Part model, mm, in its own coordinate system. Give positions to 0.01 mm unless a question says otherwise; leave off trailing zeros. Order: outer loops, then holes, each group sorted by start corner. A loop starts at its lowest first (then second) coordinate and runs counter-clockwise, first axis right, second up. Notation, with made-up numbers: (-11, 2) - (14, 2) arc R20 cw to (14, 38) - close; hole circle Ø8 at (-25.75, 89). An arc over 180 degrees is marked (long way). One line per item, written item: value.
```python
from build123d import *

# Parameters (mm, degrees)
CIRPATTERN1_COUNT = 2
CIRPATTERN1_ANGLE = 90


with BuildPart() as part:
    # BodySke → Base-Revolve (revolve)
    with BuildSketch(Plane.XY, mode=Mode.PRIVATE) as base_revolve_sk:
        Polygon((0, 0), (0, 9.15), (0.85, 9.15), (5, 5), (60, 5), (60, 0), align=None)
    revolve(base_revolve_sk.sketch.rotate(Axis((-6.35, 0, 0), (1, 0, 0)), 90), axis=Axis((-6.35, 0, 0), (1, 0, 0)))

    # Sketch3 → Cross section 0
    with BuildSketch(Plane.ZY):
        with BuildLine():
            Line((-0.99, 4.94), (0.99, 4.94))
            Line((0.99, 4.94), (0.99, -4.94))
            Line((0.99, -4.94), (-0.99, -4.94))
            Line((-0.99, -4.94), (-0.99, 4.94))
        make_face()
    # Sketch4 → Cross section 1
    with BuildSketch(Plane.ZY.offset(-5.98)):
        with BuildLine():
            Line((-0.495, 0.495), (0.495, 0.495))
            Line((0.495, 0.495), (0.495, -0.495))
            Line((0.495, -0.495), (-0.495, -0.495))
            Line((-0.495, -0.495), (-0.495, 0.495))
        make_face()
    cross = loft(mode=Mode.SUBTRACT)

    # CirPattern1: Cross ×2 about axis
    cirpattern1_axis = Axis((0, 0, 0), (1, 0, 0))
    for i in range(1, CIRPATTERN1_COUNT):
        add(cross.rotate(cirpattern1_axis, i * CIRPATTERN1_ANGLE / (CIRPATTERN1_COUNT - 1)), mode=Mode.SUBTRACT)


solid = part.part
```
1) Drop flat-ended pins along their axis: P1, Ø10, axis at x = 36.5, z = 0, coming from the +Y side; P2, Ø4, axis at x = 31.5, y = -4, coming from the -Z side; P3, Ø0.5, axis at y = 0, z = 0, coming from the -X side. Give the stop position or say it passes through.
Answer:
P1: stops at y = 5
P2: stops at z = -4.58
P3: stops at x = 5.98
2) Two-plate mould, pull along Z, no slides. Class faces 1 (the face through (5.98, 0, 0)), 2 (the face through (0, 2, -2)), 3 (the face through (33, 0, -5)): pulls with the +Z half, pulls with the -Z half, needs draft (parallel to the pull), parting line crosses it, or undercut.
Answer:
face 1: undercut
face 2: needs draft
face 3: parting line crosses it
3) Wall check: line 1 along Z through (x, y) = (55, 0.75); line 2 along Y through (x, z) = (32, 2.75); line 3 along X through (y, z) = (-0.5, 3). Give the ranges that are in metal, low to high. Write a range as [from, to].
Answer:
line 1: z = [-4.94, 4.94]
line 2: y = [-4.18, 4.18]
line 3: x = [2.61, 60]
4) Slice it at A-A on x = 28. Write the cut outline in (y, z), then the cut area to 3 significant figures.
Answer:
outline: circle Ø10 at (0, 0)
area: 78.5 mm2
